Work out the finished part from the listing and answer in its coordinate system (mm). Face numbers are marked on the shaded views. Coordinates: 2 decimals unless noted, no trailing zeros. Order: outer loops, then holes, each group sorted by start corner. A loop starts at its lowest first (then second) coordinate and runs counter-clockwise, first axis right, second up. Notation, with made-up numbers: M 75.25,64 L 85.25,64 A27 cw 85.25,83 Z; hole C -39.5,-13.75 d1. An arc over 180 degrees is marked long. Use a Markdown table: item, result.
from build123d import *

# Parameters (mm, degrees)
F1_DEPTH = 40
F2_R     = 10
F4_DEPTH = 400
F5_R     = 60.0444611856
F6_DEPTH = 30


# Not quite as in the source:
# - a fillet or chamfer that OpenCascade refuses, or shapes differently, is made with other operations: its cross-section is extruded or revolved along the edge and cut away or added


with BuildPart() as f1:
    # F0 (on Top) → F1 (new body)
    with BuildSketch(Plane.XY):
        with BuildLine():
            ThreePointArc((-260.7041027397, -159.2581299295), (-248.9883739872, -187.542401177), (-220.7041027397, -199.2581299295))
            Line((-220.7041027397, -199.2581299295), (99.2958972603, -199.2581299295))
            ThreePointArc((99.2958972603, -199.2581299295), (127.5801685078, -187.542401177), (139.2958972603, -159.2581299295))
            Line((139.2958972603, -159.2581299295), (139.2958972603, 160.7418700705))
            ThreePointArc((139.2958972603, 160.7418700705), (127.5801685078, 189.0261413179), (99.2958972603, 200.7418700705))
            Line((99.2958972603, 200.7418700705), (-220.7041027397, 200.7418700705))
            ThreePointArc((-220.7041027397, 200.7418700705), (-248.9883739872, 189.0261413179), (-260.7041027397, 160.7418700705))
            Line((-260.7041027397, 160.7418700705), (-260.7041027397, -159.2581299295))
        make_face()
    extrude(amount=F1_DEPTH)

    # F2
    f2_edges = [f1.edges().sort_by_distance(p)[0] for p in [
        (-260.704103, 0.74187, 40),
        (-248.988374, -187.542401, 40),
        (-60.704103, -199.25813, 40),
        (127.580169, -187.542401, 40),
        (139.295897, 0.74187, 40),
        (127.580169, 189.026141, 40),
        (-60.704103, 200.74187, 40),
        (-248.988374, 189.026141, 40),
    ]]
    fillet(f2_edges, radius=F2_R)

    # F3 (on face) → F4 (join)
    with BuildSketch(Plane(origin=(0, 0, 0), x_dir=(1, 0, 0), z_dir=(0, 0, -1))):
        with BuildLine():
            Line((99.2958972603, -184.0014514797), (99.2958972603, -130.7418700705))
            ThreePointArc((99.2958972603, -130.7418700705), (96.3669650722, -123.6708022586), (89.2958972603, -120.7418700705))
            Line((89.2958972603, -120.7418700705), (69.2958972603, -120.7418700705))
            ThreePointArc((69.2958972603, -120.7418700705), (62.2248294484, -123.6708022586), (59.2958972603, -130.7418700705))
            Line((59.2958972603, -130.7418700705), (59.2958972603, -184.0014514797))
            ThreePointArc((59.2958972603, -184.0014514797), (62.2248294484, -191.0725192915), (69.2958972603, -194.0014514797))
            Line((69.2958972603, -194.0014514797), (89.2958972603, -194.0014514797))
            ThreePointArc((89.2958972603, -194.0014514797), (96.3669650722, -191.0725192915), (99.2958972603, -184.0014514797))
        make_face()
        with BuildLine():
            ThreePointArc((99.2958972603, 149.2581299295), (96.3669650722, 156.3291977414), (89.2958972603, 159.2581299295))
            Line((89.2958972603, 159.2581299295), (69.2958972603, 159.2581299295))
            ThreePointArc((69.2958972603, 159.2581299295), (62.2248294484, 156.3291977414), (59.2958972603, 149.2581299295))
            Line((59.2958972603, 149.2581299295), (59.2958972603, 95.9985485203))
            ThreePointArc((59.2958972603, 95.9985485203), (62.2248294484, 88.9274807085), (69.2958972603, 85.9985485203))
            Line((69.2958972603, 85.9985485203), (89.2958972603, 85.9985485203))
            ThreePointArc((89.2958972603, 85.9985485203), (96.3669650722, 88.9274807085), (99.2958972603, 95.9985485203))
            Line((99.2958972603, 95.9985485203), (99.2958972603, 149.2581299295))
        make_face()
        with BuildLine():
            Line((-180.7041027397, 95.9985485203), (-180.7041027397, 149.2581299295))
            ThreePointArc((-180.7041027397, 149.2581299295), (-183.6330349278, 156.3291977414), (-190.7041027397, 159.2581299295))
            Line((-190.7041027397, 159.2581299295), (-210.7041027397, 159.2581299295))
            ThreePointArc((-210.7041027397, 159.2581299295), (-217.7751705516, 156.3291977414), (-220.7041027397, 149.2581299295))
            Line((-220.7041027397, 149.2581299295), (-220.7041027397, 95.9985485203))
            ThreePointArc((-220.7041027397, 95.9985485203), (-217.7751705516, 88.9274807085), (-210.7041027397, 85.9985485203))
            Line((-210.7041027397, 85.9985485203), (-190.7041027397, 85.9985485203))
            ThreePointArc((-190.7041027397, 85.9985485203), (-183.6330349278, 88.9274807085), (-180.7041027397, 95.9985485203))
        make_face()
        with BuildLine():
            Line((-180.7041027397, -184.0014514797), (-180.7041027397, -130.7418700705))
            ThreePointArc((-180.7041027397, -130.7418700705), (-183.6330349278, -123.6708022586), (-190.7041027397, -120.7418700705))
            Line((-190.7041027397, -120.7418700705), (-210.7041027397, -120.7418700705))
            ThreePointArc((-210.7041027397, -120.7418700705), (-217.7751705516, -123.6708022586), (-220.7041027397, -130.7418700705))
            Line((-220.7041027397, -130.7418700705), (-220.7041027397, -184.0014514797))
            ThreePointArc((-220.7041027397, -184.0014514797), (-217.7751705516, -191.0725192915), (-210.7041027397, -194.0014514797))
            Line((-210.7041027397, -194.0014514797), (-190.7041027397, -194.0014514797))
            ThreePointArc((-190.7041027397, -194.0014514797), (-183.6330349278, -191.0725192915), (-180.7041027397, -184.0014514797))
        make_face()
    extrude(amount=F4_DEPTH)

    # F5 (on face) → F6 (join)
    with BuildSketch(Plane.XY.offset(40)):
        Circle(F5_R)
    extrude(amount=F6_DEPTH)

    # F7: fillet of radius 50 on 1 edges, made by hand

    # F7_s1 → F7_t2 (revolve, cut)
    with BuildSketch(Plane.XZ):
        with BuildLine():
            ThreePointArc((60.0444611856, 40), (41.6048321113, 61.8330013267), (14.218704236, 70))
            Line((14.218704236, 70), (60.0444611856, 70))
            Line((60.0444611856, 70), (60.0444611856, 40))
        make_face()
    revolve(axis=Axis((0, 0, 70), (0, 0, 1)), mode=Mode.SUBTRACT)


solid = f1.part
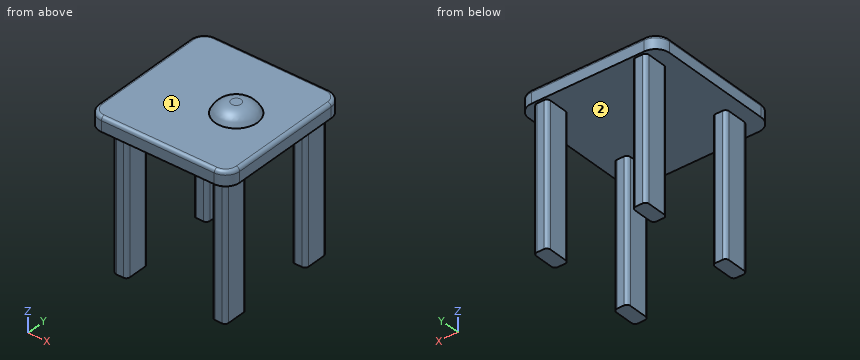
1. Section B-B on y = 90 is taken. Determine the outline of the cut face in (x, z), then the cut area to 3 significant figures.
Answers below:
| item | result |
|---|---|
| outline | M -260.7,0 L 139.3,0 L 139.3,30 A10 ccw 129.3,40 L -250.7,40 A10 ccw -260.7,30 Z |
| area | 16,000 mm² |
2. Flat-ended cylindrical pins translate along their axes: P1, Ø16, axis at y = -115.5, z = -120, coming from the +X side; P2, Ø2, axis at x = -75, y = -73, coming from the -Z side; P3, Ø6, axis at x = 82, z = -283, coming from the +Y side. Find the tip coordinate at first contact, or state that the pin passes through.
Answers below:
| item | result |
|---|---|
| P1 | x = 99.3 |
| P2 | z = 0 |
| P3 | y = 194 |
3. Find the intervals of material crossed by probe 1 along Y at (x, z) = (70.5, -316); probe 2 along Z at (x, y) = (-146.5, -128.5); probe 3 along Z at (x, y) = (65, 146), in increasing order.
Answers below:
| item | result |
|---|---|
| probe 1 | -159.26 to -86, 120.74 to 194 |
| probe 2 | 0 to 40 |
| probe 3 | -400 to 40 |
4. For a pull along X with two mould halves and no side action, classify the marked faces 1 and 2 as +X half, -X half, draft (parallel to the pull), parting line (faces both ways), or undercut.
Answers below:
| item | result |
|---|---|
| face 1 | draft |
| face 2 | undercut |
5. Section C-C on x = -81.5 is taken. Determine the outline of the cut face in (y, z), then the cut area to 3 significant figures.
Answers below:
| item | result |
|---|---|
| outline | M -199.26,0 L 200.74,0 L 200.74,30 A10 ccw 190.74,40 L -189.26,40 A10 ccw -199.26,30 Z |
| area | 16,000 mm² |
6. Section A-A on z = -28.5 is taken. Give the number of separate pieces and of enclosed holes in the cut face, then the cut area to 3 significant figures.
Answers below:
| item | result |
|---|---|
| separate pieces | 4 |
| enclosed holes | 0 |
| area | 11,400 mm² |
